The model under review builds one solid part; all positions refer to its coordinate system, in mm. Face numbers are marked on the shaded views. A direction names the side the tool comes from. Round coordinates to 2 decimals unless told otherwise and drop trailing zeros. Order: outer loops, then holes, each group sorted by start corner. A loop starts at its lowest first (then second) coordinate and runs counter-clockwise, first axis right, second up. Notation, with made-up numbers: M -10,-1 L 33,-1 A15 ccw 33,26 Z; hole C 58,34.25 d2. An arc over 180 degrees is marked long. Answer as a JSON object with one key per item and string values. Group by question number.
1. Add section C-C on z = 41.5. State the section outline as (x, y) points, and give its area (3 significant figures).
2. To check wall thickness, follow probe 1 along Z at (x, y) = (0, 4); probe 2 along X at (y, z) = (-1, 120.5); probe 3 along Z at (x, y) = (12, 10). State the ranges of each line that lie inside material, in increasing order. Write a range as [from, to].
3. Machinability: for the marked faces 1 and 2, which of the approach directions +Z, -Z, +X, -X, +Y, -Y give a long, thin tool a straight path to every point of the face, cutting with its end or side? Answer none if there is none.
4. Add section B-B on z = -31.5. State the section outline as (x, y) points.
5. Clearance check with flat-ended pins moving along their axes: P1, Ø4, axis at x = -18.5, z = -127, coming from the +Y side; P2, Ø5, axis at x = -4, z = 100, coming from the +Y side; P3, Ø2, axis at x = -2.5, y = 28, coming from the +Z side; P4, Ø5, axis at y = 13, z = -124.5, coming from the -X side. State where each tip first meets the part, or that it passes through.
6. Add section A-A on x = 0. State the section outline as (y, z) points.
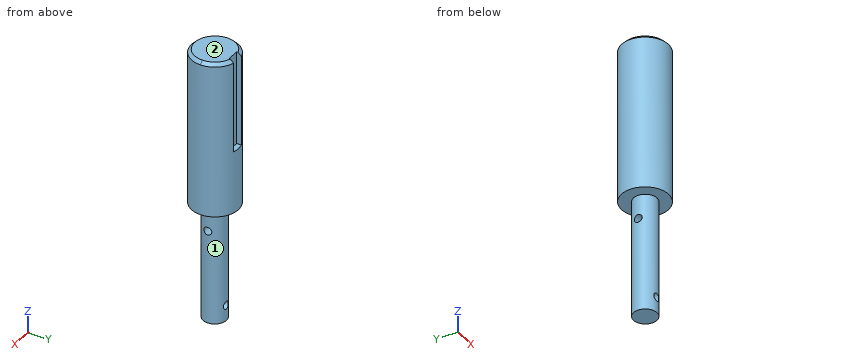
```python
from build123d import *

# Parameters (mm, degrees)
SKETCH1_R               = 15
BOSS_EXTRUDE1_DEPTH     = 100
SKETCH2_W               = 8
SKETCH2_H               = 7
CUT_EXTRUDE1_DEPTH      = 60
CHAMFER1_SIZE           = 2
SCALE1_SCALE            = 2
SKETCH3_R               = 15
BOSS_EXTRUDE2_DEPTH     = 150
SKETCH4_R               = 5
CUT_EXTRUDE2_DEPTH      = 31.301047562
CUT_EXTRUDE2_DEPTH_BACK = 30.698952438
SKETCH5_R               = 5
CUT_EXTRUDE3_DEPTH      = 31
CUT_EXTRUDE3_DEPTH_BACK = 31


with BuildPart() as part:
    # Sketch1 → Boss-Extrude1 (new body)
    with BuildSketch(Plane.XY):
        Circle(SKETCH1_R)
    extrude(amount=BOSS_EXTRUDE1_DEPTH)

    # Sketch2 → Cut-Extrude1 (cut)
    with BuildSketch(Plane.XY.offset(100)):
        with Locations((0, 15)):
            Rectangle(SKETCH2_W, SKETCH2_H)
    extrude(amount=-CUT_EXTRUDE1_DEPTH, mode=Mode.SUBTRACT)

    # Chamfer1
    chamfer1_edges = [part.edges().sort_by_distance(p)[0] for p in [
        (-9.082951062, -11.937336386, 100),
    ]]
    chamfer(chamfer1_edges, length=CHAMFER1_SIZE)


with BuildPart() as part_1:
    # Scale1: scaled about (0, -0.301047562, 49.420279713)
    add(part.part.scale(SCALE1_SCALE).moved(Location((0, 0.301047562, -49.420279713))))

    # Sketch3 → Boss-Extrude2 (add)
    with BuildSketch(Plane(origin=(0, 0, -49.420279708), x_dir=(-1, 0, 0), z_dir=(0, 0, -1))):
        Circle(SKETCH3_R)
    extrude(amount=BOSS_EXTRUDE2_DEPTH)

    # Sketch4 → Cut-Extrude2 (cut, two sides)
    with BuildSketch(Plane(origin=(0, 0, 0), x_dir=(1, 0, 0), z_dir=(0, 1, 0))) as cut_extrude2_sk:
        with Locations((0, 179.420279708)):
            Circle(SKETCH4_R)
    extrude(amount=CUT_EXTRUDE2_DEPTH, mode=Mode.SUBTRACT)
    extrude(cut_extrude2_sk.sketch, amount=-CUT_EXTRUDE2_DEPTH_BACK, mode=Mode.SUBTRACT)

    # Sketch5 → Cut-Extrude3 (cut, two sides)
    with BuildSketch(Plane(origin=(0, 0, 0), x_dir=(0, 0, -1), z_dir=(1, 0, 0))) as cut_extrude3_sk:
        with Locations((79.420279708, 0)):
            Circle(SKETCH5_R)
    extrude(amount=CUT_EXTRUDE3_DEPTH, mode=Mode.SUBTRACT)
    extrude(cut_extrude3_sk.sketch, amount=-CUT_EXTRUDE3_DEPTH_BACK, mode=Mode.SUBTRACT)


solid = part_1.part
```
Recorded:
{
 "1": {"outline": "M -8,23.3 L -8,29.21 A30 ccw long 8,29.21 L 8,23.3 Z", "area": "2,720 mm²"},
 "2": {"probe 1": "z = [-199.42, -184.42], [-174.42, -82.42], [-76.42, 150.58]", "probe 2": "x = [-29.97, 29.97]", "probe 3": "z = [-49.42, 150.58]"},
 "3": {"face 1": "-Z", "face 2": "+Z, +X, -X, +Y, -Y"},
 "4": {"outline": "C 0,0.3 d60"},
 "5": {"P1": "passes through", "P2": "stops at y = 23.3", "P3": "stops at z = 30.58", "P4": "stops at x = -10.71"},
 "6": {"outline": "M -29.7,-49.42 L -15,-49.42 L -15,-174.42 L 15,-174.42 L 15,-49.42 L 30.3,-49.42 L 30.3,30.58 L 23.3,30.58 L 23.3,150.58 L -25.7,150.58 L -29.7,146.58 Z; M -15,-199.42 L 15,-199.42 L 15,-184.42 L -15,-184.42 Z; hole C 0,-79.42 d10"}
}
